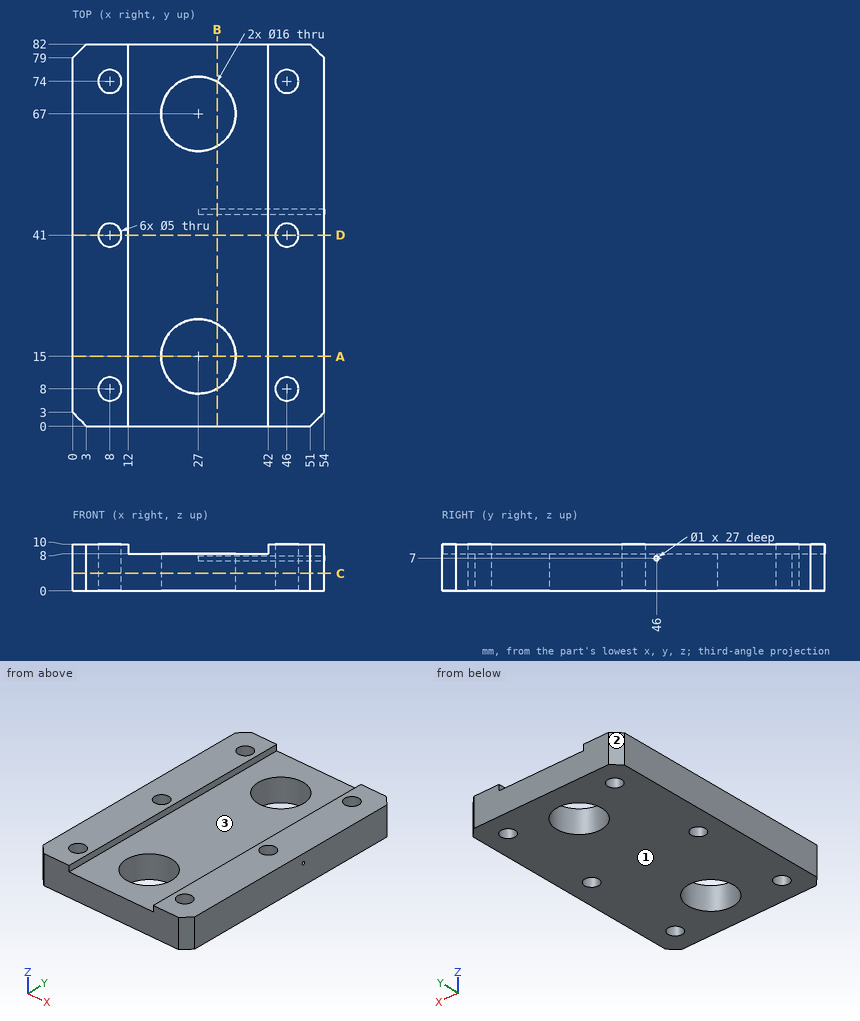
Study the drawing (mm; zero at the part's minimum x, y, z) and answer. Give positions to 0.01 mm unless a question says otherwise; leave off trailing zeros. Order: outer loops, then holes, each group sorted by start corner. A loop starts at its lowest first (then second) coordinate and runs counter-clockwise, first axis right, second up. Notation, with made-up numbers: (16, -39.75) -> (58, -39.75) arc R14 ccw to (58, -30.75) -> close; hole circle Ø1 at (65.5, 26.25). An arc over 180 degrees is marked (long way). Put each result on its own line as item: value.
Item 1: A cutting plane is placed at B-B on x = 31. Give the vertices of the cut face in (y, z).
Established:
outline: (0, 0) -> (8.07, 0) -> (8.07, 8) -> (0, 8) -> close; (21.93, 0) -> (60.07, 0) -> (60.07, 8) -> (21.93, 8) -> close; (73.93, 0) -> (82, 0) -> (82, 8) -> (73.93, 8) -> close; hole circle Ø1 at (46, 7)
Item 2: A cutting plane is placed at C-C on z = 3.75. Count the separate pieces of the cut face and the enclosed holes in it, plus the area to 3 significant figures.
Established:
separate pieces: 1
enclosed holes: 8
area: 3,890 mm^2
Item 3: A cutting plane is placed at D-D on y = 41. Give the vertices of the cut face in (x, z), plus the area to 3 significant figures.
Established:
outline: (0, 0) -> (5.5, 0) -> (5.5, 10) -> (0, 10) -> close; (10.5, 0) -> (43.5, 0) -> (43.5, 10) -> (42, 10) -> (42, 8) -> (12, 8) -> (12, 10) -> (10.5, 10) -> close; (48.5, 0) -> (54, 0) -> (54, 10) -> (48.5, 10) -> close
area: 380 mm^2
Item 4: A cutting plane is placed at A-A on y = 15. Give the vertices of the cut face in (x, z).
Established:
outline: (0, 0) -> (19, 0) -> (19, 8) -> (12, 8) -> (12, 10) -> (0, 10) -> close; (35, 0) -> (54, 0) -> (54, 10) -> (42, 10) -> (42, 8) -> (35, 8) -> close
Item 5: For a pull along X with two mould halves and no side action, classify the marked faces 1, 2 and 3 as released by +X, released by -X, zero draft, split by the parting line, or undercut.
Established:
face 1: zero draft
face 2: released by -X
face 3: undercut
Item 6: Given P1, Ø2, axis at x = 33.5, y = 68.5, coming from the -Z side; P2, Ø1.5, axis at x = 40.5, y = 19.5, coming from the +Z side; P3, Ø24, axis at x = 32.5, y = 51.5, coming from the +Z side; P4, Ø0.8, axis at y = 46, z = 7, coming from the +X side, each flat-ended and moving along its own axis, determine where each tip first touches the part or whether it passes through.
Established:
P1: passes through
P2: stops at z = 8
P3: stops at z = 10
P4: stops at x = 27
Item 7: Straight lines are drawn through the part: line 1 (Y direction, x = 46, z = 2.5); line 2 (Y direction, x = 26.5, z = 1.25); line 3 (Z direction, x = 38.5, y = 14). For each, find the intervals that lie inside material, in ascending order.
Established:
line 1: y = 0 to 5.5, 10.5 to 38.5, 43.5 to 71.5, 76.5 to 82
line 2: y = 0 to 7.02, 22.98 to 59.02, 74.98 to 82
line 3: z = 0 to 8
